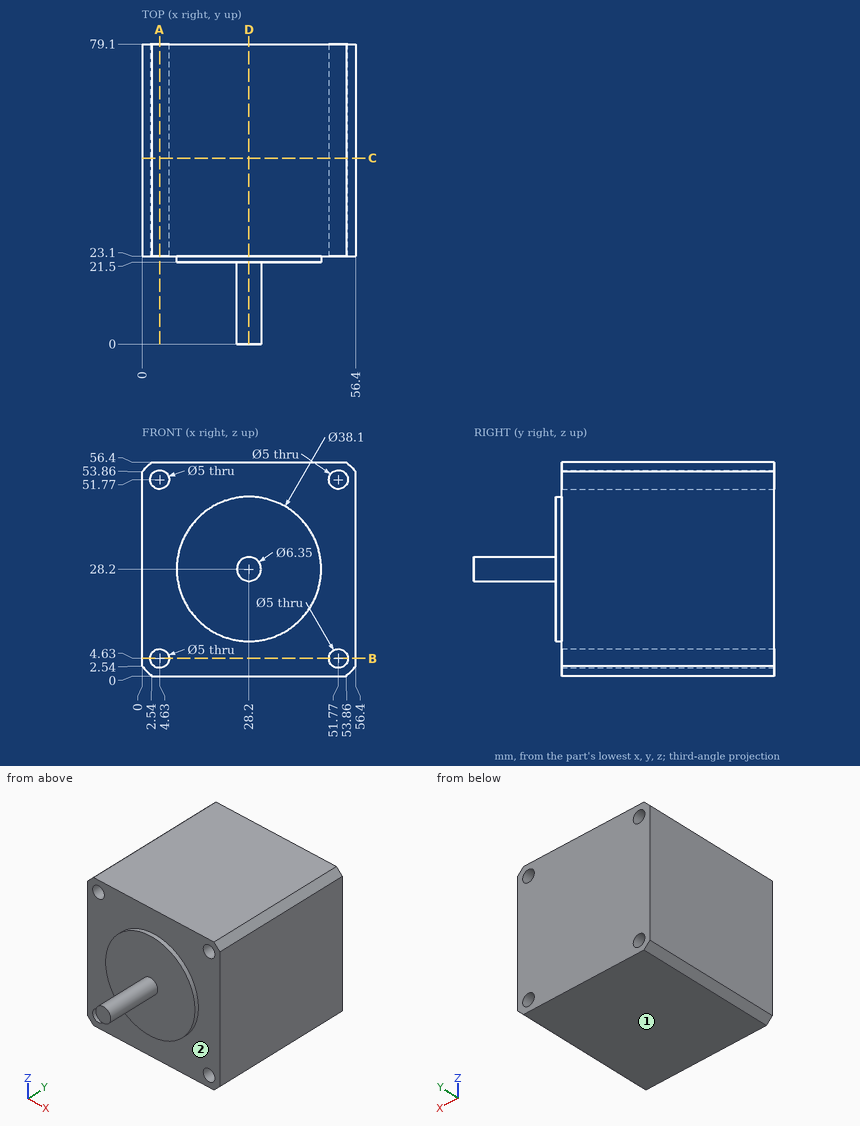
Check sheet for the drawn part. Datum: minimum x, y, z corner. Units: mm. A direction names the side the tool comes from. Round coordinates to 2 decimals unless told otherwise and drop trailing zeros. Write each loop counter-clockwise with the first axis right and the second up, starting at its lowest first coordinate (ties: lowest second). Pieces come first, ordered by that corner, then holes. Notation, with made-up numbers: (-13, 87) -> (-4, 87) arc R17 ccw to (-4, 110) -> close; hole circle Ø9 at (48, 39). An arc over 180 degrees is marked (long way). One line per item, written item: value. Start each with the question number.
(1) Cross-section at B-B, the plane z = 4.63. Record the cut outline in (x, y), and give its area (3 significant figures).
(2) Cross-section at D-D, the plane x = 28.2. Record the cut outline in (y, z) (3 decimals).
(3) Access from +Z, -Z, +X, -X, +Y, -Y to the whole of each face (thin tool, end or side, straight path). Record for the marked faces 1 and 2.
(4) Scan lines: line 1 (Z direction, x = 4.63, y = 36); line 2 (Z direction, x = 51, y = 63). Record each from-to range of solid material in increasing order. Write a range as [from, to].
(5) Cross-section at A-A, the plane x = 4.63. Record the cut outline in (y, z), and give its area (3 significant figures).
(6) Cross-section at C-C, the plane y = 49. Record the cut outline in (x, z).
(7) Go/stop test with flat-tipped pins: pin 1 Ø4 at (y, z) = (17, 22.5) entering from +X; pin 2 Ø2 at (x, z) = (42.5, 9.5) entering from -Y. Record where each tip stops, or that it passes through.
Answer:
1. outline: (0, 23.1) -> (2.13, 23.1) -> (2.13, 79.1) -> (0, 79.1) -> close; (7.13, 23.1) -> (49.27, 23.1) -> (49.27, 79.1) -> (7.13, 79.1) -> close; (54.27, 23.1) -> (56.4, 23.1) -> (56.4, 79.1) -> (54.27, 79.1) -> close
1. area: 2,600 mm²
2. outline: (0, 25.025) -> (21.5, 25.025) -> (21.5, 9.15) -> (23.1, 9.15) -> (23.1, 0) -> (79.1, 0) -> (79.1, 56.4) -> (23.1, 56.4) -> (23.1, 47.25) -> (21.5, 47.25) -> (21.5, 31.375) -> (0, 31.375) -> close
3. face 1: -Z, +X, -X, +Y, -Y
3. face 2: -Y
4. line 1: [0, 2.13], [7.13, 49.27], [54.27, 56.4]
4. line 2: [0, 2.25], [7.01, 49.39], [54.15, 56.4]
5. outline: (23.1, 0) -> (79.1, 0) -> (79.1, 2.13) -> (23.1, 2.13) -> close; (23.1, 7.13) -> (79.1, 7.13) -> (79.1, 49.27) -> (23.1, 49.27) -> close; (23.1, 54.27) -> (79.1, 54.27) -> (79.1, 56.4) -> (23.1, 56.4) -> close
5. area: 2,600 mm²
6. outline: (0, 2.54) -> (2.54, 0) -> (53.86, 0) -> (56.4, 2.54) -> (56.4, 53.86) -> (53.86, 56.4) -> (2.54, 56.4) -> (0, 53.86) -> close; hole circle Ø5 at (4.63, 4.63); hole circle Ø5 at (4.63, 51.77); hole circle Ø5 at (51.77, 4.63); hole circle Ø5 at (51.77, 51.77)
7. pin 1: through
7. pin 2: y = 23.1
